Geometry: final body of the model. Coordinates: model frame, mm. Give positions to 0.01 mm unless a question says otherwise; leave off trailing zeros. Order: outer loops, then holes, each group sorted by start corner. A loop starts at its lowest first (then second) coordinate and runs counter-clockwise, first axis right, second up. Notation, with made-up numbers: M -24.75,75.25 L -6.75,75.25 A8 cw -6.75,85.25 Z; hole C -11.75,-3 d2. An arc over 180 degrees is marked long. One line per item, written item: value. Start each with the question number.
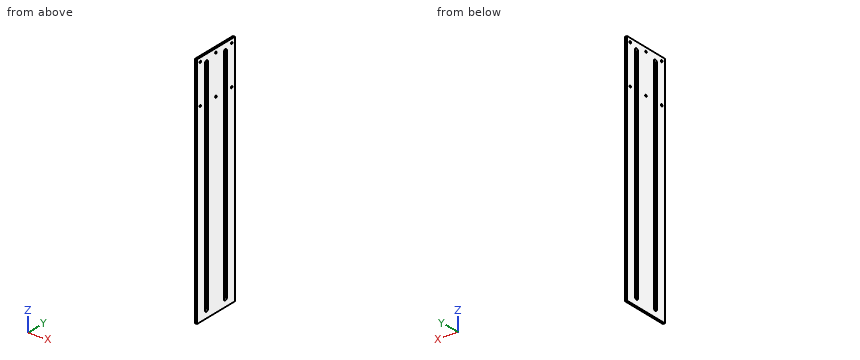
```python
from build123d import *

# Parameters (mm, degrees)
SKETCH1_W         = 381
SKETCH1_H         = 76.2
OUTER_CUT_DEPTH   = 1.5875
SLOTS_DEPTH       = 195.298586266
SKETCH3_R         = 1.5875
MOUNT_HOLES_DEPTH = 195.298586266


with BuildPart() as part:
    # Sketch1 → Outer Cut (new, symmetric)
    with BuildSketch(Plane(origin=(0, 0, 0), x_dir=(0, 0, -1), z_dir=(1, 0, 0))):
        Rectangle(SKETCH1_W, SKETCH1_H)
    extrude(amount=OUTER_CUT_DEPTH, both=True)

    # Sketch2 → Slots (cut, through all)
    with BuildSketch(Plane(origin=(1.5875, 0, 0), x_dir=(0, 0, -1), z_dir=(1, 0, 0))):
        with BuildLine():
            Line((-177.8, 22.225), (177.8, 22.225))
            ThreePointArc((177.8, 22.225), (180.975, 19.05), (177.8, 15.875))
            Line((177.8, 15.875), (-177.8, 15.875))
            ThreePointArc((-177.8, 15.875), (-180.975, 19.05), (-177.8, 22.225))
        make_face()
        with BuildLine():
            Line((-177.8, -22.225), (177.8, -22.225))
            ThreePointArc((177.8, -22.225), (180.975, -19.05), (177.8, -15.875))
            Line((177.8, -15.875), (-177.8, -15.875))
            ThreePointArc((-177.8, -15.875), (-180.975, -19.05), (-177.8, -22.225))
        make_face()
    extrude(amount=-SLOTS_DEPTH, mode=Mode.SUBTRACT)

    # Sketch3 → Mount Holes (cut, through all)
    with BuildSketch(Plane(origin=(1.5875, 0, 0), x_dir=(0, 0, -1), z_dir=(1, 0, 0))):
        with Locations((-184.15, 31.75)):
            Circle(SKETCH3_R)
        with Locations((-120.65, 31.75)):
            Circle(SKETCH3_R)
        with Locations(Location((-120.65, -31.75, 0), (0, 0, 180))):
            Circle(SKETCH3_R)
        with Locations(Location((-184.15, -31.75, 0), (0, 0, 180))):
            Circle(SKETCH3_R)
        with Locations((-184.15, 0)):
            Circle(SKETCH3_R)
        with Locations((-120.65, 0)):
            Circle(SKETCH3_R)
    extrude(amount=-MOUNT_HOLES_DEPTH, mode=Mode.SUBTRACT)


solid = part.part
```
Q1. Ray query, line 1 along Y through (x, z) = (1.05, 71) (3 decimals); line 2 along Y through (x, z) = (-0.1, 120.65) (1 decimal); line 3 along Z through (x, y) = (-0.75, 18). Return the intervals inside material, ascending. Write a range as [from, to].
Q2. Section query C-C on x = -0.5. Give the number of separate pieces and of enclosed holes in the cut face, and give its area (3 significant figures).
Q3. Section query B-B on z = -95.5. Return loops of the section in (x, y) (1 decimal), and give its area (3 significant figures).
Q4. Section query D-D on y = -19. Return loops of the section in (x, z).
Q5. Contact query for a flat-ended pin moving along its axis: pin 1 (5 mm diameter, centred on y = 31.75, z = 184.15, fed in from -X). Output: stop coordinate, or through.
Q6. Section query A-A on y = 19.05. Return loops of the section in (x, z) (1 decimal).
Results below:
1. line 1: [-38.1, -22.225], [-15.875, 15.875], [22.225, 38.1]
1. line 2: [-38.1, -33.3], [-30.2, -22.2], [-15.9, -1.6], [1.6, 15.9], [22.2, 30.2], [33.3, 38.1]
1. line 3: [-190.5, -180.8], [180.8, 190.5]
2. separate pieces: 1
2. enclosed holes: 8
2. area: 24,400 mm2
3. outline: M -1.6,-38.1 L 1.6,-38.1 L 1.6,-22.2 L -1.6,-22.2 Z; M -1.6,-15.9 L 1.6,-15.9 L 1.6,15.9 L -1.6,15.9 Z; M -1.6,22.2 L 1.6,22.2 L 1.6,38.1 L -1.6,38.1 Z
3. area: 202 mm2
4. outline: M -1.59,-190.5 L 1.59,-190.5 L 1.59,-180.97 L -1.59,-180.97 Z; M -1.59,180.97 L 1.59,180.97 L 1.59,190.5 L -1.59,190.5 Z
5. pin 1: x = -1.59
6. outline: M -1.6,-190.5 L 1.6,-190.5 L 1.6,-181 L -1.6,-181 Z; M -1.6,181 L 1.6,181 L 1.6,190.5 L -1.6,190.5 Z
